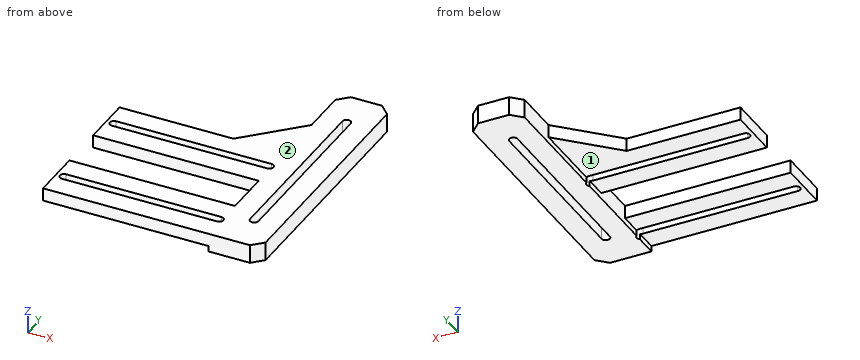
```python
from build123d import *

# Parameters (mm, degrees)
SKETCH_1_W                  = 20
SKETCH_1_H                  = 20
SKETCH_1_W_2                = 64
SKETCH_1_H_2                = 18
SKETCH_1_H_3                = 42
EXTRUDE_1_DEPTH             = 5
SKETCH_2_W                  = 20
SKETCH_2_H                  = 100
EXTRUDE_2_DEPTH             = 2.2
HOLE_START                  = -2.2
HOLE_WIZARD_3_2_3_2_1_DEPTH = 7.2
HOLE_WIZARD_3_2_3_2_2_DEPTH = 7.2
RIB_1_REACH                 = 88.214
SKETCH_11_WALL_W            = 202.712111226
SKETCH_11_WALL_H            = 5
CHAMFER_1_SIZE              = 4


# Read off the part's stored shape, not the designer's step: Ø3.2 (3.2) 直径槽口1, Ø3.2 (3.2) 直径槽口2
with BuildPart() as part:
    # 草图1 → 凸台-拉伸1 (new body)
    with BuildSketch(Plane.XY):
        with Locations((45, -24)):
            Rectangle(SKETCH_1_W, SKETCH_1_H)
        with Locations((3, -24)):
            Rectangle(SKETCH_1_W_2, SKETCH_1_H)
        with Locations((3, 14)):
            Rectangle(SKETCH_1_W_2, SKETCH_1_H)
        with Locations((45, -5)):
            Rectangle(SKETCH_1_W, SKETCH_1_H_2)
        with Locations((45, 45)):
            Rectangle(SKETCH_1_W, SKETCH_1_H_3)
        with Locations((45, 14)):
            Rectangle(SKETCH_1_W, SKETCH_1_H)
    extrude(amount=EXTRUDE_1_DEPTH)

    # 草图2 → 凸台-拉伸2 (add)
    with BuildSketch(Plane(origin=(0, 0, 0), x_dir=(-1, 0, 0), z_dir=(0, 0, -1))):
        with Locations((-45, 16)):
            Rectangle(SKETCH_2_W, SKETCH_2_H)
    extrude(amount=EXTRUDE_2_DEPTH)

    # Ø3.2 (3.2) 直径槽口1 outline → Ø3.2 (3.2) 直径槽口1 (cut)
    with BuildSketch(Plane.XY.offset(HOLE_START)):
        with BuildLine():
            Line((34, -22.4), (-26, -22.4))
            ThreePointArc((-26, -22.4), (-27.6, -24), (-26, -25.6))
            Line((-26, -25.6), (34, -25.6))
            ThreePointArc((34, -25.6), (35.6, -24), (34, -22.4))
        make_face()
        with BuildLine():
            ThreePointArc((34, 12.4), (35.6, 14), (34, 15.6))
            Line((34, 15.6), (-26, 15.6))
            ThreePointArc((-26, 15.6), (-27.6, 14), (-26, 12.4))
            Line((-26, 12.4), (34, 12.4))
        make_face()
    extrude(amount=HOLE_WIZARD_3_2_3_2_1_DEPTH, mode=Mode.SUBTRACT)

    # Ø3.2 (3.2) 直径槽口2 outline → Ø3.2 (3.2) 直径槽口2 (cut)
    with BuildSketch(Plane.XY.offset(HOLE_START)):
        with BuildLine():
            Line((46.6, -19), (46.6, 51))
            ThreePointArc((46.6, 51), (45, 52.6), (43.4, 51))
            Line((43.4, 51), (43.4, -19))
            ThreePointArc((43.4, -19), (45, -20.6), (46.6, -19))
        make_face()
    extrude(amount=HOLE_WIZARD_3_2_3_2_2_DEPTH, mode=Mode.SUBTRACT)

    # 草图11 wall → 筋1 (add, up to next)
    with BuildSketch(Plane(origin=(25, 34, 5), x_dir=(0.707106781187, 0.707106781187, 0), z_dir=(-0.707106781187, 0.707106781187, 0)), mode=Mode.PRIVATE) as rib_1_sk1:
        with Locations((0, 2.5)):
            Rectangle(SKETCH_11_WALL_W, SKETCH_11_WALL_H)
    rib_1_tool1 = extrude(rib_1_sk1.sketch, amount=-RIB_1_REACH, mode=Mode.PRIVATE) - part.part
    add(rib_1_tool1.solids().sort_by_distance((25, 34, 5))[0])

    # 倒角1
    chamfer_1_edges = [part.edges().sort_by_distance(p)[0] for p in [
        (35, 66, 1.4),
        (55, 66, 1.4),
        (55, -34, 1.4),
    ]]
    chamfer(chamfer_1_edges, length=CHAMFER_1_SIZE)


solid = part.part
```
Source: CAD feature listing. Evaluate the final solid. Frame: model axes, mm. Face numbers are marked on the shaded views. A direction names the side the tool comes from. Give positions to 0.01 mm unless a question says otherwise; leave off trailing zeros. Order: outer loops, then holes, each group sorted by start corner. A loop starts at its lowest first (then second) coordinate and runs counter-clockwise, first axis right, second up. Notation, with made-up numbers: (20.5, 36.5) -> (68.5, 36.5) arc R13 ccw to (68.5, 55.5) -> close; hole circle Ø9 at (3.5, -24.75). An arc over 180 degrees is marked (long way). Use a Markdown table: item, result.
Q1. Material intervals for line 1 (Y direction, x = -7.5, z = 3); line 2 (X direction, y = 4.5, z = 4.25); line 3 (X direction, y = 47, z = -0.5), sorted ascending. Write a range as [from, to].
A:
| item | result |
|---|---|
| line 1 | [-34, -25.6], [-22.4, -14], [4, 12.4], [15.6, 24] |
| line 2 | [-29, 43.4], [46.6, 55] |
| line 3 | [35, 43.4], [46.6, 55] |
Q2. Section D-D (x = 45). Return the cut outline in (y, z), and give its area (3 significant figures).
A:
| item | result |
|---|---|
| outline | (-34, -2.2) -> (-20.6, -2.2) -> (-20.6, 5) -> (-34, 5) -> close; (52.6, -2.2) -> (66, -2.2) -> (66, 5) -> (52.6, 5) -> close |
| area | 193 mm^2 |
Q3. Section C-C (y = 14). Return the cut outline in (x, z).
A:
| item | result |
|---|---|
| outline | (-29, 0) -> (-27.6, 0) -> (-27.6, 5) -> (-29, 5) -> close; (35.6, -2.2) -> (43.4, -2.2) -> (43.4, 5) -> (35.6, 5) -> close; (46.6, -2.2) -> (55, -2.2) -> (55, 5) -> (46.6, 5) -> close |
Q4. Section B-B (x = 23.5). Return the cut outline in (y, z), and give its area (4 significant figures).
A:
| item | result |
|---|---|
| outline | (-34, 0) -> (-25.6, 0) -> (-25.6, 5) -> (-34, 5) -> close; (-22.4, 0) -> (-14, 0) -> (-14, 5) -> (-22.4, 5) -> close; (4, 0) -> (12.4, 0) -> (12.4, 5) -> (4, 5) -> close; (15.6, 0) -> (32.5, 0) -> (32.5, 5) -> (15.6, 5) -> close |
| area | 210.5 mm^2 |
Q5. Access query for the marked faces 1 and 2. Directions: +Z, -Z, +X, -X, +Y, -Y. A direction counts if a zero-diameter tool reaches every point of the face in a straight line with its end or side. Return the directions, or none.
A:
| item | result |
|---|---|
| face 1 | -Z, -X, +Y, -Y |
| face 2 | +Z, +X, -X, +Y, -Y |
Q6. First-contact query: P1, Ø6, axis at x = 14.5, y = -23.5, coming from the -Z side; P2, Ø4, axis at x = 1, z = 3, coming from the +Y side; P3, Ø1.8, axis at y = -30.5, z = -1, coming from the -X side. Flat tips, straight axial feed; report the tip coordinate or a pass-through.
A:
| item | result |
|---|---|
| P1 | z = 0 |
| P2 | y = 24 |
| P3 | x = 35 |
Q7. Section A-A (z = 3.75). Return the cut outline in (x, y).
A:
| item | result |
|---|---|
| outline | (-29, -34) -> (51, -34) -> (55, -30) -> (55, 62) -> (51, 66) -> (39, 66) -> (35, 62) -> (35, 44) -> (15, 24) -> (-29, 24) -> (-29, 4) -> (35, 4) -> (35, -14) -> (-29, -14) -> close; hole (-26, -25.6) -> (34, -25.6) arc R1.6 ccw to (34, -22.4) -> (-26, -22.4) arc R1.6 ccw to start; hole (-26, 12.4) -> (34, 12.4) arc R1.6 ccw to (34, 15.6) -> (-26, 15.6) arc R1.6 ccw to start; hole (43.4, -19) arc R1.6 ccw to (46.6, -19) -> (46.6, 51) arc R1.6 ccw to (43.4, 51) -> close |
